The model under review builds one solid part; all positions refer to its coordinate system, in mm. A direction names the side the tool comes from. Round coordinates to 2 decimals unless told otherwise and drop trailing zeros. Write each loop counter-clockwise with the first axis right and the second up, starting at its lowest first coordinate (ties: lowest second). Pieces come first, ordered by that corner, then holes. Notation, with made-up numbers: (45.5, -4) -> (69.5, -4) arc R25 cw to (69.5, 29) -> close; hole circle Ø10 at (6.25, -38). An arc over 180 degrees is marked (long way). Answer in a Markdown table with one row per item. Add a question column.
```python
from build123d import *

# Parameters (mm, degrees)
F1_DEPTH = 0.5


with BuildPart() as f1:
    # F0 (on Front) → F1 (new body)
    with BuildSketch(Plane.XZ):
        with BuildLine():
            ThreePointArc((2.954972, -2.626698), (3.591449, -3.001585), (4.240578, -2.649057))
            ThreePointArc((4.240578, -2.649057), (0, 5), (-4.240578, -2.649057))
            ThreePointArc((-4.240578, -2.649057), (-3.591449, -3.001585), (-2.954972, -2.626698))
            Line((-2.954972, -2.626698), (-2.298715, -1.490027))
            ThreePointArc((-2.298715, -1.490027), (-2.232321, -1.264386), (-2.276439, -1.033356))
            ThreePointArc((-2.276439, -1.033356), (-2.443471, -0.528631), (-2.5, 0))
            ThreePointArc((-2.5, 0), (-2.646447, 0.353553), (-3, 0.5))
            Line((-3, 0.5), (-3.614208, 0.5))
            ThreePointArc((-3.614208, 0.5), (-4.012119, 0.697235), (-4.096102, 1.133333))
            ThreePointArc((-4.096102, 1.133333), (-3.257408, 2.729797), (-1.832226, 3.834768))
            ThreePointArc((-1.832226, 3.834768), (-1.468558, 3.861178), (-1.183657, 3.633619))
            Line((-1.183657, 3.633619), (-0.586866, 2.599947))
            ThreePointArc((-0.586866, 2.599947), (-0.480462, 2.500497), (-0.336691, 2.477224))
            ThreePointArc((-0.336691, 2.477224), (0, 2.5), (0.336691, 2.477224))
            ThreePointArc((0.336691, 2.477224), (0.480462, 2.500497), (0.586866, 2.599947))
            Line((0.586866, 2.599947), (1.183657, 3.633619))
            ThreePointArc((1.183657, 3.633619), (1.468558, 3.861178), (1.832226, 3.834768))
            ThreePointArc((1.832226, 3.834768), (3.257408, 2.729797), (4.096102, 1.133333))
            ThreePointArc((4.096102, 1.133333), (4.012119, 0.697235), (3.614208, 0.5))
            Line((3.614208, 0.5), (3, 0.5))
            ThreePointArc((3, 0.5), (2.646447, 0.353553), (2.5, 0))
            ThreePointArc((2.5, 0), (2.443471, -0.528631), (2.276439, -1.033356))
            ThreePointArc((2.276439, -1.033356), (2.232321, -1.264386), (2.298715, -1.490027))
            Line((2.298715, -1.490027), (2.954972, -2.626698))
        make_face()
    extrude(amount=F1_DEPTH)


solid = f1.part
```
1. Add section A-A on y = -0.1. Write out the cut boundary in (x, z).
2. Mouldability with a two-part tool opening along X and no side actions: class faces 3 (the flat face through (0, 0, 3)), 4 (the cylindrical face through (-3.274, -0.246, 2.71)), 5 (the cylindrical face through (0.1, -0.2, 5)) as pulls with the +X half, pulls with the -X half, needs draft (parallel to the pull), parting line crosses it, or undercut.
3. Tool access review of faces 1 (the flat face through (0, -0.5, 3)), 2 (the cylindrical face through (3.24, -0.25, 2.75)): name each direction out of +Z, -Z, +X, -X, +Y, -Y from which nothing blocks a thin tool from reaching the whole face with its end or side.
4. For L1, parallel to X at y = -0.3, z = 3.25; L2, parallel to X at y = -0.15, z = 3; L3, parallel to X at y = -0.3, z = 4, list the stretches that pass through material, from the lowest coordinate up.
5. Add section D-D on x = 0. Write out the cut boundary in (y, z), plus the area to 3 significant figures.
6. Add section C-C on z = 2.75. Write out the cut boundary in (x, y).
7. Add section B-B on z = 1.25. Write out the cut boundary in (x, y).
Filled in:
| question | item | result |
|---|---|---|
| 1 | outline | (-4.24, -2.65) arc R0.75 ccw to (-2.95, -2.63) -> (-2.3, -1.49) arc R0.5 ccw to (-2.28, -1.03) arc R2.5 cw to (-2.5, 0) arc R0.5 ccw to (-3, 0.5) -> (-3.61, 0.5) arc R0.5 cw to (-4.1, 1.13) arc R4.25 cw to (-1.83, 3.83) arc R0.5 cw to (-1.18, 3.63) -> (-0.59, 2.6) arc R0.25 ccw to (-0.34, 2.48) arc R2.5 cw to (0.34, 2.48) arc R0.25 ccw to (0.59, 2.6) -> (1.18, 3.63) arc R0.5 cw to (1.83, 3.83) arc R4.25 cw to (4.1, 1.13) arc R0.5 cw to (3.61, 0.5) -> (3, 0.5) arc R0.5 ccw to (2.5, 0) arc R2.5 cw to (2.28, -1.03) arc R0.5 ccw to (2.3, -1.49) -> (2.95, -2.63) arc R0.75 ccw to (4.24, -2.65) arc R5 ccw (long way) to start |
| 2 | face 3 | needs draft |
| 2 | face 4 | undercut |
| 2 | face 5 | parting line crosses it |
| 3 | face 1 | +Z, -Z, +X, -X, -Y |
| 3 | face 2 | +Y, -Y |
| 4 | L1 | -3.8 to -2.74, -0.96 to 0.96, 2.74 to 3.8 |
| 4 | L2 | -4 to -3.01, -0.82 to 0.82, 3.01 to 4 |
| 4 | L3 | -3 to 3 |
| 5 | outline | (-0.5, 2.5) -> (0, 2.5) -> (0, 5) -> (-0.5, 5) -> close |
| 5 | area | 1.25 mm² |
| 6 | outline | (-4.18, -0.5) -> (-3.24, -0.5) -> (-3.24, 0) -> (-4.18, 0) -> close; (-0.67, -0.5) -> (0.67, -0.5) -> (0.67, 0) -> (-0.67, 0) -> close; (3.24, -0.5) -> (4.18, -0.5) -> (4.18, 0) -> (3.24, 0) -> close |
| 7 | outline | (-4.84, -0.5) -> (-4.06, -0.5) -> (-4.06, 0) -> (-4.84, 0) -> close; (4.06, -0.5) -> (4.84, -0.5) -> (4.84, 0) -> (4.06, 0) -> close |
